Input: dimensioned drawing with shaded views. Units: mm. Origin: part minimum x, y, z. A direction names the side the tool comes from. Give positions to 0.01 mm unless a question says otherwise; leave off trailing zeros. Loops run counter-clockwise (first coordinate to the right, second up) from the corner with the lowest first, then second, coordinate; pieces in that order, holes last. Notation, with made-up numbers: M -1.75,-21.75 L 53.25,-21.75 A16 ccw 53.25,-14.75 Z; hole C 48.5,71 d1. An arc over 180 degrees is marked long. Answer in a Markdown table with one row per item.
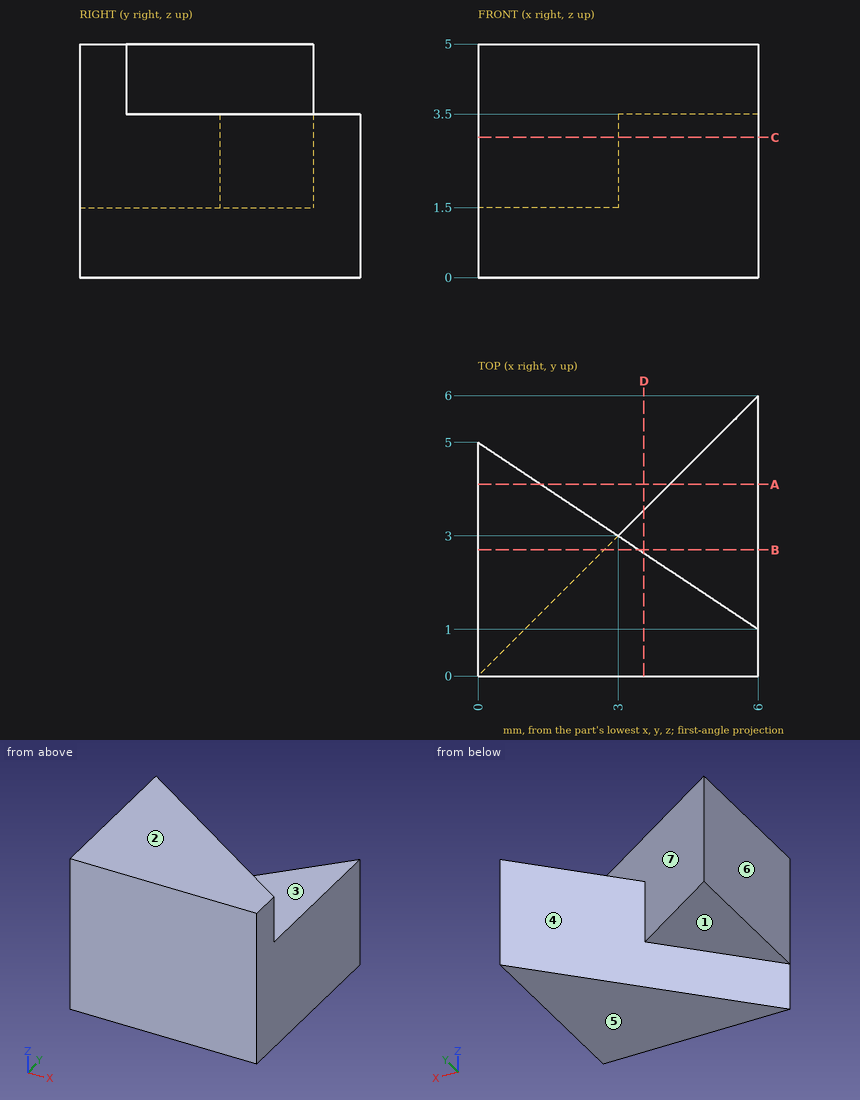
Q1. Ray query, probe 1 along Z at (x, y) = (4.95, 1.75); probe 2 along Z at (x, y) = (1.9, 2.45); probe 3 along X at (y, z) = (4.05, 3.7) (3 decimals). Return the intervals inside material, ascending. Write a range as from..to.
Values follow:
| item | result |
|---|---|
| probe 1 | 0..3.5 |
| probe 2 | 1.5..5 |
| probe 3 | 0..1.425 |
Q2. Reachability of the marked faces 1, 2 and 3 from +Z, -Z, +X, -X, +Y, -Y: full face, straight path, thin tool, end or side. Return the list, or none.
Values follow:
| item | result |
|---|---|
| face 1 | -Z, -X, +Y |
| face 2 | +Z, +X, -X, +Y, -Y |
| face 3 | +Z, +X, +Y |
Q3. Section query B-B (y = 2.7). Output: boundary loops of the cut face in (x, z), plus the area to 3 significant figures.
Values follow:
| item | result |
|---|---|
| outline | M 0,1.5 L 2.7,1.5 L 2.7,0 L 6,0 L 6,3.5 L 3.45,3.5 L 3.45,5 L 0,5 Z |
| area | 22.1 mm^2 |
Q4. Mould query, pull axis X, two halves, no side actions, for the marked faces 4, 5, 6 and 7. Classes: +X half, -X half, draft (parallel to the pull), parting line (faces both ways), or undercut.
Values follow:
| item | result |
|---|---|
| face 4 | undercut |
| face 5 | draft |
| face 6 | -X half |
| face 7 | undercut |
Q5. Section query D-D (x = 3.55). Output: boundary loops of the cut face in (y, z), plus the area to 3 significant figures.
Values follow:
| item | result |
|---|---|
| outline | M 0,0 L 3.55,0 L 3.55,3.5 L 2.63,3.5 L 2.63,5 L 0,5 Z |
| area | 16.4 mm^2 |
Q6. Section query C-C (z = 3). Output: boundary loops of the cut face in (x, y).
Values follow:
| item | result |
|---|---|
| outline | M 0,0 L 6,0 L 6,6 L 3,3 L 0,5 Z |
Q7. Contact query for flat-ended pins moving along their axis: pin 1 Ø0.9 at (x, y) = (1.5, 3) entering from -Z; pin 2 Ø2 at (x, y) = (2, 5) entering from -Z. Output: stop coordinate, or through.
Values follow:
| item | result |
|---|---|
| pin 1 | z = 1.5 |
| pin 2 | through |
Q8. Section query A-A (y = 4.1). Output: boundary loops of the cut face in (x, z), plus the area to 3 significant figures.
Values follow:
| item | result |
|---|---|
| outline | M 0,1.5 L 1.35,1.5 L 1.35,5 L 0,5 Z; M 4.1,0 L 6,0 L 6,3.5 L 4.1,3.5 Z |
| area | 11.4 mm^2 |
